Work out the finished part from the listing and answer in its coordinate system (mm). A direction names the side the tool comes from. Round coordinates to 2 decimals unless told otherwise and drop trailing zeros. Loops run counter-clockwise (first coordinate to the right, second up) from the corner with the lowest first, then second, coordinate; pieces in that order, holes last. Notation, with made-up numbers: (47.25, 48) -> (93.25, 48) arc R31 cw to (93.25, 78) -> close; hole circle Ø9 at (60.5, 45). An arc over 180 degrees is marked (long way). Use CSV: the item, a comma, the result in double quotes. Start each with the question number.
from build123d import *

# Parameters (mm, degrees)
F0_W     = 20.32
F0_H     = 12.7
F0_R     = 1.8415
F1_DEPTH = 6.096
F2_W     = 6.096
F2_H     = 27.94
F3_DEPTH = 19.812
F4_R     = 1.614101
F5_DEPTH = 25.4


with BuildPart() as f1:
    # F0 (on Top) → F1 (new body)
    with BuildSketch(Plane.XY):
        with Locations((10.16, 6.35)):
            Rectangle(F0_W, F0_H)
        with Locations((3.81, 5.08)):
            Circle(F0_R, mode=Mode.SUBTRACT)
        with Locations((13.462, 5.08)):
            Circle(F0_R, mode=Mode.SUBTRACT)
    extrude(amount=F1_DEPTH)

    # F2 (on face) → F3 (join)
    with BuildSketch(Plane.XY.offset(6.096)):
        with Locations((23.368, 5.08)):
            Rectangle(F2_W, F2_H)
    extrude(amount=-F3_DEPTH)

    # F4 (on face) → F5 (cut)
    with BuildSketch(Plane(origin=(20.32, 0, 0), x_dir=(0, -1, 0), z_dir=(-1, 0, 0))):
        with Locations((5.08, -5.461)):
            Circle(F4_R)
        with Locations((-4.5339, -5.461)):
            Circle(F4_R)
        with Locations((-14.1478, -5.461)):
            Circle(F4_R)
    extrude(amount=-F5_DEPTH, mode=Mode.SUBTRACT)


solid = f1.part
Q1. Section A-A, the plane y = -5.08 is taken. Write down the section's boundary in (x, z).
Q2. Straight lines are drawn through the part: line 1 (Y direction, x = 3.81, z = 4.75); line 2 (Y direction, x = 23.5, z = -5.75); line 3 (Z direction, x = 24.75, y = -5.08). For each, find the intervals that lie inside material, in ascending order. Write a range as from..to.
Q3. For a pull along X with two mould halves and no side action, classify faces 1 (the flat face through (26.416, 4.9, -3.7)), 2 (the cylindrical face through (2.45, 6.32, 3.01)), 3 (the cylindrical face through (11.622, 5.161, 3.005)), 4 (the flat face through (23, -8.89, -4)) as pulls with the +X half, pulls with the -X half, needs draft (parallel to the pull), parting line crosses it, or undercut.
Q4. Section B-B, the plane x = 3.81 is taken. Write down the section's boundary in (y, z).
Q5. Section D-D, the plane y = 4.5 is taken. Write down the section's boundary in (x, z), and give its area (3 significant figures).
Q6. Each of these flat-tipped pins is pushed along its axis until it touches: pin 1 (3 mm diameter, centred on x = 13, z = 4, fed in from -Y); pin 2 (10 mm diameter, centred on y = 12, z = -8.5, fed in from -X); pin 3 (10 mm diameter, centred on x = 8, y = 7.5, fed in from -Z); pin 4 (1.9 mm diameter, centred on y = -5.08, z = -5.461, fed in from -X). Where does it stop, or does it pass through?
Q7. Section C-C, the plane z = 1.75 is taken. Write down the section's boundary in (x, y), and give its area (3 significant figures).
Q8. Which of the six approach directions +Z, -Z, +X, -X, +Y, -Y give full straight-line access (tool end or side, diameter ignored) to faces 5 (the flat face through (10, 6, 0)), 6 (the flat face through (10, 12.7, 3)), 7 (the flat face through (10, 0, 3)), 8 (the flat face through (23, 19.05, -4))?
Report:
1,outline,"(20.32, -13.72) -> (26.42, -13.72) -> (26.42, -7.08) -> (20.32, -7.08) -> close; (20.32, -3.85) -> (26.42, -3.85) -> (26.42, 6.1) -> (20.32, 6.1) -> close"
2,line 1,"y = 0..3.24, 6.92..12.7"
2,line 2,"y = -8.89..-6.67, -3.49..2.95, 6.12..12.56, 15.74..19.05"
2,line 3,"z = -13.72..-7.08, -3.85..6.1"
3,face 1,"pulls with the +X half"
3,face 2,"undercut"
3,face 3,"undercut"
3,face 4,"needs draft"
4,outline,"(0, 0) -> (3.24, 0) -> (3.24, 6.1) -> (0, 6.1) -> close; (6.92, 0) -> (12.7, 0) -> (12.7, 6.1) -> (6.92, 6.1) -> close"
5,outline,"(0, 0) -> (2.06, 0) -> (2.06, 6.1) -> (0, 6.1) -> close; (5.56, 0) -> (11.71, 0) -> (11.71, 6.1) -> (5.56, 6.1) -> close; (15.21, 0) -> (20.32, 0) -> (20.32, -3.85) -> (26.42, -3.85) -> (26.42, 6.1) -> (15.21, 6.1) -> close; (20.32, -13.72) -> (26.42, -13.72) -> (26.42, -7.07) -> (20.32, -7.07) -> close"
5,area,"182 mm²"
6,pin 1,"stops at y = 0"
6,pin 2,"stops at x = 20.32"
6,pin 3,"stops at z = 0"
6,pin 4,"passes through"
7,outline,"(0, 0) -> (20.32, 0) -> (20.32, -8.89) -> (26.42, -8.89) -> (26.42, 19.05) -> (20.32, 19.05) -> (20.32, 12.7) -> (0, 12.7) -> close; hole circle Ø3.68 at (3.81, 5.08); hole circle Ø3.68 at (13.46, 5.08)"
7,area,"407 mm²"
8,face 5,"-Z, -X, +Y, -Y"
8,face 6,"+Z, -Z, -X, +Y"
8,face 7,"+Z, -Z, -X, -Y"
8,face 8,"+Z, -Z, +X, -X, +Y"
